Read the model definition and answer for the solid it produces. Units are mm, in the model's axes. Face numbers are marked on the shaded views. A direction names the side the tool comes from. Coordinates: 2 decimals unless noted, no trailing zeros. Order: outer loops, then holes, each group sorted by start corner. A loop starts at its lowest first (then second) coordinate and runs counter-clockwise, first axis right, second up. Notation, with made-up numbers: M 18.5,77.25 L 26.5,77.25 A37 ccw 26.5,114.25 Z; hole C -26,15 d4. An arc over 180 degrees is marked long. Put each result on its own line as item: value.
Autodesk Inventor part; units mm, degrees
ref_plane "YZ Plane" through (0, 0, 0) normal (1, 0, 0) x (0, 1, 0)
ref_plane "XZ Plane" through (0, 0, 0) normal (0, 1, 0) x (-1, 0, 0)
ref_plane "XY Plane" through (0, 0, 0) normal (0, 0, 1) x (1, 0, 0)
sketch "Esquisse1" plane through (0, 0, 0) normal (0, 0, 1) x (1, 0, 0)
  line L0 (0, 0) -> (-118.5, 0)
  line L1 (-118.5, 0) -> (-118.5, -425)
  line L2 (-118.5, -425) -> (0, -425)
  line L3 (0, -425) -> (0, 0)
  dimension "d0" = 425
  dimension "d3" = 118.5
extrude "Extrusion1" add sketch "Esquisse1" along normal blind 18.55
sketch "Esquisse2" plane through (0, 0, 18.55) normal (0, 0, 1) x (1, 0, 0)
  line L0 (-118.5, 0) -> (-118.5, -425) construction
  line L1 (-118.5, -50) -> (-99.95, -50)
  line L2 (-99.95, -50) -> (-99.95, -150)
  line L3 (-99.95, -150) -> (-118.5, -150)
  line L4 (-118.5, -150) -> (-118.5, -50)
  line L5 (-118.5, -250) -> (-99.95, -250)
  line L6 (-99.95, -250) -> (-99.95, -350)
  line L7 (-99.95, -350) -> (-118.5, -350)
  line L8 (-118.5, -350) -> (-118.5, -250)
  line L9 (0, 0) -> (-118.5, 0)
  line L10 (-118.5, -425) -> (0, -425)
  line L11 (-59.25, 0) -> (-59.25, -425) construction
  line L12 (0, 0) -> (0, -425) construction
  line L13 (0, -50) -> (-18.55, -50)
  line L14 (-18.55, -50) -> (-18.55, -150)
  line L15 (-18.55, -150) -> (0, -150)
  line L16 (0, -150) -> (0, -50)
  line L17 (0, -250) -> (-18.55, -250)
  line L18 (-18.55, -250) -> (-18.55, -350)
  line L19 (-18.55, -350) -> (0, -350)
  line L20 (0, -350) -> (0, -250)
  dimension "d27" = 18.55
  dimension "d28" = 100
  dimension "d29" = 100
  dimension "d30" = 100
  dimension "d31" = 50
  dimension "d32" = 75
extrude "Extrusion2" cut sketch "Esquisse2" against normal blind 18.55
sketch "Esquisse3" plane through (0, 0, 18.55) normal (0, 0, 1) x (1, 0, 0)
  line L0 (0, -425) -> (0, 0)
  line L1 (-118.5, -425) -> (0, -425)
  line L2 (-118.5, -350) -> (-118.5, -425)
  line L3 (-67.5329, -385) -> (-63.4915, -378)
  line L4 (-63.4915, -378) -> (-55.4085, -378)
  line L5 (-55.4085, -378) -> (-51.3671, -385)
  line L6 (-51.3671, -385) -> (-55.4085, -392)
  line L7 (-55.4085, -392) -> (-63.4915, -392)
  line L8 (-63.4915, -392) -> (-67.5329, -385)
  line L9 (-99.95, -250) -> (-99.95, -350)
  line L10 (-18.55, -350) -> (-18.55, -250)
  line L11 (-55.4085, -207) -> (-63.4915, -207)
  line L12 (-63.4915, -207) -> (-67.5329, -200)
  line L13 (-67.5329, -200) -> (-63.4915, -193)
  line L14 (-63.4915, -193) -> (-55.4085, -193)
  line L15 (-55.4085, -193) -> (-51.3671, -200)
  line L16 (-51.3671, -200) -> (-55.4085, -207)
  line L17 (-118.5, -150) -> (-118.5, -250)
  line L18 (-118.5, -200) -> (-59.45, -200) construction
  point P0 (-59.45, -385)
  dimension "d43" = 14
  dimension "d44" = 40.5
  dimension "d45" = 40.9
  dimension "d46" = 40
extrude "Extrusion3" cut sketch "Esquisse3" against normal blind 7
sketch "Esquisse4" plane through (0, 0, 18.55) normal (0, 0, 1) x (1, 0, 0)
  circle A0 centre (-101.0725, -51.1225) radius 1.5875
  circle A1 centre (-17.4275, -51.1225) radius 1.5875
  circle A2 centre (-101.0725, -148.8775) radius 1.5875
  circle A3 centre (-17.4275, -148.8775) radius 1.5875
  line L0 (-118.5, -50) -> (-99.95, -50)
  line L1 (-99.95, -50) -> (-101.0725, -51.1225) construction
  line L2 (-99.95, -150) -> (-99.95, -50)
  line L3 (-101.0725, -148.8775) -> (-99.95, -150) construction
  line L4 (-99.95, -150) -> (-118.5, -150)
  line L5 (-18.55, -50) -> (0, -50)
  line L6 (-18.55, -50) -> (-17.4275, -51.1225) construction
  line L7 (-18.55, -150) -> (-18.55, -50)
  line L8 (-18.55, -150) -> (-17.4275, -148.8775) construction
  line L9 (0, -150) -> (-18.55, -150)
  line L10 (-118.5, -150) -> (-118.5, -250)
  line L11 (-118.5, -200) -> (0, -200) construction
  line L12 (0, -250) -> (0, -150)
  circle A4 centre (-101.0725, -348.8775) radius 1.5875
  circle A5 centre (-17.4275, -348.8775) radius 1.5875
  circle A6 centre (-101.0725, -251.1225) radius 1.5875
  circle A7 centre (-17.4275, -251.1225) radius 1.5875
  line L13 (-99.95, -350) -> (-101.0725, -348.8775) construction
  line L14 (-101.0725, -251.1225) -> (-99.95, -250) construction
  line L15 (-18.55, -350) -> (-17.4275, -348.8775) construction
  line L16 (-18.55, -250) -> (-17.4275, -251.1225) construction
  point P0 (0, 0)
  point P1 (-99.95, -350)
  point P2 (-99.95, -250)
  point P3 (-18.55, -350)
  point P4 (-18.55, -250)
  dimension "d34" = 3.175
  dimension "d51" = 45
  dimension "d52" = 45
  dimension "d53" = 45
  dimension "d54" = 45
extrude "Extrusion4" cut sketch "Esquisse4" against normal blind 18.55
sketch "Esquisse5" plane through (0, 0, 18.55) normal (0, 0, 1) x (1, 0, 0)
  circle A0 centre (-110.3475, -25) radius 2.25
  circle A1 centre (-110.3475, -180) radius 2.25
  circle A2 centre (-110.3475, -395) radius 2.25
  line L0 (-118.5, -50) -> (-102.1951, -50)
  line L1 (-110.3475, -50) -> (-110.3475, -425) construction
  line L2 (-118.5, -425) -> (0, -425)
  line L3 (-110.3475, -50) -> (-110.3475, 0) construction
  line L4 (0, 0) -> (-118.5, 0)
  line L5 (-99.95, -350) -> (-118.5, -350)
  line L6 (-102.1951, -150) -> (-118.5, -150)
  line L7 (-59.25, 0) -> (-59.25, -425) construction
  circle A3 centre (-8.1525, -25) radius 2.25
  circle A4 centre (-8.1525, -180) radius 2.25
  circle A5 centre (-8.1525, -395) radius 2.25
  line L8 (0, -50) -> (-16.3049, -50)
  line L9 (-8.1525, -50) -> (-8.1525, -425) construction
  line L10 (-8.1525, -50) -> (-8.1525, 0) construction
  line L11 (-16.9625, -350.1) -> (0, -350)
  line L12 (-16.3049, -150) -> (0, -150)
  circle A6 centre (-110.3475, -220) radius 2.25
  line L13 (-118.5, -250) -> (-102.1951, -250)
  circle A7 centre (-8.1525, -220) radius 2.25
  point P0 (-101.5375, -350.1)
  dimension "d37" = 4.5
  dimension "d38" = 30
  dimension "d39" = 45
  dimension "d40" = 30
  dimension "d56" = 30
extrude "Extrusion5" cut sketch "Esquisse5" against normal blind 120
sketch "Esquisse6" plane through (0, 0, 11.55) normal (0, 0, 1) x (1, 0, 0)
  circle A0 centre (-59.45, -385) radius 5.25
  line L0 (-63.4915, -392) -> (-67.5329, -385)
  line L1 (-63.4915, -378) -> (-55.4085, -378)
  line L2 (-63.4915, -392) -> (-55.4085, -378) construction
  line L3 (-63.4915, -378) -> (-55.4085, -392) construction
  circle A1 centre (-59.45, -200) radius 5.25
  line L4 (-63.4915, -193) -> (-55.4085, -207) construction
  point P0 (0, 0)
  dimension "d47" = 10.5
extrude "Extrusion6" cut sketch "Esquisse6" against normal blind 18
sketch "Esquisse7" plane through (0, 0, 0) normal (0, 0, -1) x (-1, 0, 0)
  circle A0 centre (59.45, -200) radius 5.25 construction
  circle A1 centre (59.45, -200) radius 30
  circle A2 centre (59.45, -385) radius 5.25 construction
  circle A3 centre (59.45, -385) radius 30
  point P0 (0, 0)
  dimension "d57" = 60
extrude "Extrusion7" cut sketch "Esquisse7" against normal blind 2.5
properties part number "rail"
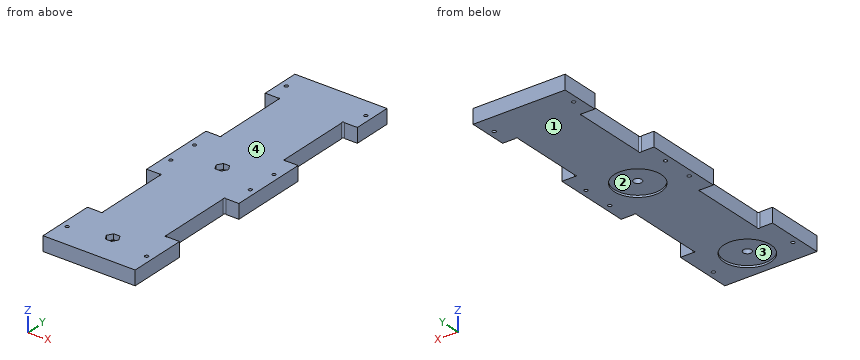
Q1. Find section D-D on y = -102. Write down the section's boundary in (x, z), plus the area to 3 significant figures.
Answers below:
outline: M -99.95,0 L -18.55,0 L -18.55,18.55 L -99.95,18.55 Z
area: 1,510 mm^2
Q2. Find section C-C on z = 5.5. Give the number of separate pieces and of enclosed holes in the cut face, plus the area to 3 significant figures.
Answers below:
separate pieces: 1
enclosed holes: 10
area: 42,600 mm^2
Q3. A tool of negligible diameter and unlimited length cuts with its end or side. For the marked faces 3 and 4, from which of +Z, -Z, +X, -X, +Y, -Y can it reach the whole face along a straight path? Write none if from no direction.
Answers below:
face 3: -Z
face 4: +Z, +X, -X, +Y, -Y
Q4. For a pull along Y with two mould halves and no side action, classify the marked faces 1 and 2 as +Y half, -Y half, draft (parallel to the pull), parting line (faces both ways), or undercut.
Answers below:
face 1: draft
face 2: undercut
Q5. Find section B-B on x = -80.5. Write down the section's boundary in (y, z).
Answers below:
outline: M -425,0 L -406.38,0 L -406.38,2.5 L -363.62,2.5 L -363.62,0 L -221.38,0 L -221.38,2.5 L -178.62,2.5 L -178.62,0 L 0,0 L 0,18.55 L -425,18.55 Z
Q6. Consider line 1 along Y through (x, z) = (-59.45, 5.75); line 2 along X through (y, z) = (-220, 4.25); line 3 along Y through (x, z) = (-106.5, 13). Determine where each line is inside the solid, lowest interval first.
Answers below:
line 1: y = -425 to -390.25, -379.75 to -205.25, -194.75 to 0
line 2: x = -118.5 to -112.6, -108.1 to -10.4, -5.9 to 0
line 3: y = -425 to -350, -250 to -150, -50 to 0
Q7. Given pin 1 (6 mm diameter, centred on x = -8.15, y = -180, fed in from -Z); pin 2 (5.5 mm diameter, centred on y = -300, z = 11, fed in from +X); pin 3 (18 mm diameter, centred on x = -46, y = -199, fed in from -Z); pin 4 (10 mm diameter, centred on y = -324, z = 14.5, fed in from -X), each flat-ended and moving along its own axis, determine where each tip first touches the part or whether it passes through.
Answers below:
pin 1: stops at z = 0
pin 2: stops at x = -18.55
pin 3: stops at z = 2.5
pin 4: stops at x = -99.95
Q8. Find section A-A on x = -59.45. Write down the section's boundary in (y, z).
Answers below:
outline: M -425,0 L -415,0 L -415,2.5 L -390.25,2.5 L -390.25,11.55 L -392,11.55 L -392,18.55 L -425,18.55 Z; M -379.75,2.5 L -355,2.5 L -355,0 L -230,0 L -230,2.5 L -205.25,2.5 L -205.25,11.55 L -207,11.55 L -207,18.55 L -378,18.55 L -378,11.55 L -379.75,11.55 Z; M -194.75,2.5 L -170,2.5 L -170,0 L 0,0 L 0,18.55 L -193,18.55 L -193,11.55 L -194.75,11.55 Z
